Verification items for the finished model (mm, model axes). Face numbers are marked on the shaded views. A direction names the side the tool comes from. Coordinates: 2 decimals unless noted, no trailing zeros. Write each loop counter-clockwise with the first axis right and the second up, starting at its lowest first coordinate (ties: lowest second). Pieces come first, ordered by that corner, then holes. Notation, with made-up numbers: (8, -12.75) -> (12, -12.75) arc R14 cw to (12, 7.25) -> close; hole circle Ø7 at (64, -19). An arc over 180 degrees is marked (long way). Answer in a Markdown table with one row per item.
```python
from build123d import *

# Parameters (mm, degrees)
SKETCH1_R           = 40
SKETCH1_R_2         = 6
SKETCH1_W           = 6.8
SKETCH1_H           = 1.7
BOSS_EXTRUDE1_DEPTH = 10
SKETCH3_R           = 40
SKETCH3_W           = 30
SKETCH3_H           = 46.499999994
BOSS_EXTRUDE3_DEPTH = 25
CUT_EXTRUDE1_START  = -35
CUT_EXTRUDE1_DEPTH  = 35
SKETCH5_R           = 2.55
CUT_EXTRUDE2_DEPTH  = 5
CUT_EXTRUDE3_DEPTH  = 25
SKETCH8_W           = 22
SKETCH8_H           = 8
CUT_EXTRUDE4_DEPTH  = 22


with BuildPart() as part:
    # Sketch1 → Boss-Extrude1 (new body)
    with BuildSketch(Plane.XY):
        with Locations((0, 222.499999997)):
            Circle(SKETCH1_R)
        with Locations((0, 234.5)):
            Circle(SKETCH1_R_2, mode=Mode.SUBTRACT)
        with Locations((0, 200.1)):
            Rectangle(SKETCH1_W, SKETCH1_H, mode=Mode.SUBTRACT)
        with BuildLine():
            ThreePointArc((11, 243.75), (9.75, 242.5), (11, 241.25))
            ThreePointArc((11, 241.25), (12.25, 242.5), (11, 243.75))
        make_face(mode=Mode.SUBTRACT)
        with BuildLine():
            ThreePointArc((-11, 241.25), (-9.75, 242.5), (-11, 243.75))
            ThreePointArc((-11, 243.75), (-12.25, 242.5), (-11, 241.25))
        make_face(mode=Mode.SUBTRACT)
        with BuildLine():
            ThreePointArc((11, 201.25), (12.25, 202.5), (11, 203.75))
            ThreePointArc((11, 203.75), (9.75, 202.5), (11, 201.25))
        make_face(mode=Mode.SUBTRACT)
        with BuildLine():
            ThreePointArc((-11, 201.25), (-9.75, 202.5), (-11, 203.75))
            ThreePointArc((-11, 203.75), (-12.25, 202.5), (-11, 201.25))
        make_face(mode=Mode.SUBTRACT)
    extrude(amount=BOSS_EXTRUDE1_DEPTH)

    # Sketch3 → Boss-Extrude3 (add)
    with BuildSketch(Plane.XY.offset(10)):
        with Locations((0, 222.499999997)):
            Circle(SKETCH3_R)
        with Locations((0, 222.499999997)):
            Rectangle(SKETCH3_W, SKETCH3_H, mode=Mode.SUBTRACT)
    extrude(amount=BOSS_EXTRUDE3_DEPTH)

    # Sketch4 → Cut-Extrude1 (cut)
    with BuildSketch(Plane.XY.offset(35).offset(CUT_EXTRUDE1_START)):
        with BuildLine():
            ThreePointArc((40, 222.499999997), (38.912456167, 231.763949212), (35.708962247, 240.524150885))
            ThreePointArc((35.708962247, 240.524150885), (31.77566454, 233.14486234), (30.74061322, 224.84706751))
            ThreePointArc((30.74061322, 224.84706751), (30.809531665, 222.499999997), (30.74061322, 220.152932484))
            ThreePointArc((30.74061322, 220.152932484), (31.77566454, 211.855137653), (35.708962247, 204.475849108))
            ThreePointArc((35.708962247, 204.475849108), (38.912456167, 213.236050782), (40, 222.499999997))
        make_face()
        with BuildLine():
            ThreePointArc((-2.347067513, 191.759386777), (-10.644862344, 190.724335457), (-18.024150889, 186.79103775))
            ThreePointArc((-18.024150889, 186.79103775), (0, 182.499999997), (18.024150889, 186.79103775))
            ThreePointArc((18.024150889, 186.79103775), (10.644862344, 190.724335457), (2.347067513, 191.759386777))
            ThreePointArc((2.347067513, 191.759386777), (0, 191.690468331), (-2.347067513, 191.759386777))
        make_face()
        with BuildLine():
            ThreePointArc((18.024150889, 258.208962244), (0, 262.499999997), (-18.024150889, 258.208962244))
            ThreePointArc((-18.024150889, 258.208962244), (-10.644862344, 254.275664537), (-2.347067513, 253.240613217))
            ThreePointArc((-2.347067513, 253.240613217), (0, 253.309531662), (2.347067513, 253.240613217))
            ThreePointArc((2.347067513, 253.240613217), (10.644862344, 254.275664537), (18.024150889, 258.208962244))
        make_face()
        with BuildLine():
            ThreePointArc((-30.74061322, 220.152932484), (-30.809531665, 222.499999997), (-30.74061322, 224.84706751))
            ThreePointArc((-30.74061322, 224.84706751), (-31.77566454, 233.14486234), (-35.708962247, 240.524150885))
            ThreePointArc((-35.708962247, 240.524150885), (-40, 222.499999997), (-35.708962247, 204.475849108))
            ThreePointArc((-35.708962247, 204.475849108), (-31.77566454, 211.855137653), (-30.74061322, 220.152932484))
        make_face()
    extrude(amount=CUT_EXTRUDE1_DEPTH, mode=Mode.SUBTRACT)

    # Sketch5 → Cut-Extrude2 (cut)
    with BuildSketch(Plane.XY.offset(35)):
        with Locations((-22.627416998, 245.127416995)):
            Circle(SKETCH5_R)
        with Locations(Location((22.627416998, 245.127416995, 0), (0, 0, 180))):
            Circle(SKETCH5_R)
        with Locations((22.627416998, 199.872582999)):
            Circle(SKETCH5_R)
        with Locations(Location((-22.627416998, 199.872582999, 0), (0, 0, 180))):
            Circle(SKETCH5_R)
    extrude(amount=-CUT_EXTRUDE2_DEPTH, mode=Mode.SUBTRACT)

    # Sketch6 → Cut-Extrude3 (cut)
    with BuildSketch(Plane.XY.offset(35)):
        with BuildLine():
            Line((-15, 218.499999997), (-15, 226.499999997))
            ThreePointArc((-15, 226.499999997), (-19, 222.499999997), (-15, 218.499999997))
        make_face()
        with BuildLine():
            Line((15, 218.499999997), (15, 226.499999997))
            ThreePointArc((15, 226.499999997), (19, 222.499999997), (15, 218.499999997))
        make_face()
    extrude(amount=-CUT_EXTRUDE3_DEPTH, mode=Mode.SUBTRACT)

    # Sketch8 → Cut-Extrude4 (cut)
    with BuildSketch(Plane(origin=(-15, 0, 0), x_dir=(0, 0, -1), z_dir=(1, 0, 0))):
        with Locations((-11, 222.499999997)):
            Rectangle(SKETCH8_W, SKETCH8_H)
    extrude(amount=-CUT_EXTRUDE4_DEPTH, mode=Mode.SUBTRACT)


solid = part.part
```
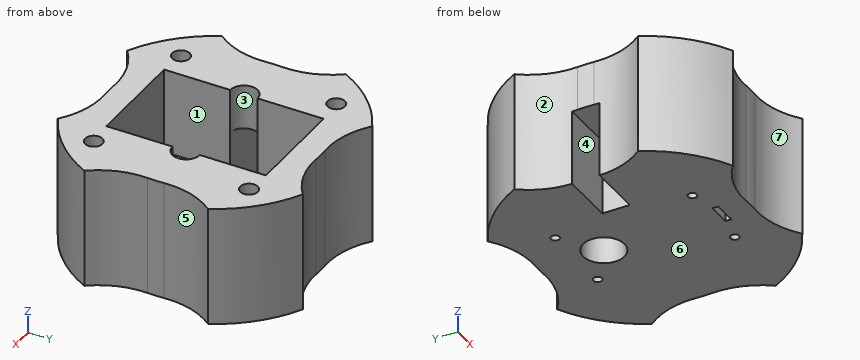
1. Go/stop test with flat-tipped pins: pin 1 (15.5 mm diameter, centred on y = 213, z = 24.5, fed in from +X); pin 2 (6 mm diameter, centred on y = 202.5, z = 20.5, fed in from +X); pin 3 (1.9 mm diameter, centred on y = 200, z = 5.5, fed in from +X). Record where each tip stops, or that it passes through.
Findings below:
| item | result |
|---|---|
| pin 1 | stops at x = 35.12 |
| pin 2 | stops at x = 35.71 |
| pin 3 | stops at x = 33.7 |
2. Sectioned sample at D-D, the plane z = 14.5. Record the cut outline in (x, y).
Findings below:
| item | result |
|---|---|
| outline | (-35.71, 204.48) arc R40 ccw to (-18.02, 186.79) arc R23 cw to (-2.35, 191.76) arc R40 ccw to (2.35, 191.76) arc R23 cw to (18.02, 186.79) arc R40 ccw to (35.71, 204.48) arc R23 cw to (30.74, 220.15) arc R40 ccw to (30.74, 224.85) arc R23 cw to (35.71, 240.52) arc R40 ccw to (18.02, 258.21) arc R23 cw to (2.35, 253.24) arc R40 ccw to (-2.35, 253.24) arc R23 cw to (-18.02, 258.21) arc R40 ccw to (-35.71, 240.52) arc R23 cw to (-30.7, 226.5) -> (-15, 226.5) -> (-15, 245.75) -> (15, 245.75) -> (15, 226.5) arc R4 cw to (15, 218.5) -> (15, 199.25) -> (-15, 199.25) -> (-15, 218.5) -> (-30.7, 218.5) arc R23 cw to start |
3. Sectioned sample at B-B, the plane z = 29. Record the cut outline in (x, y).
Findings below:
| item | result |
|---|---|
| outline | (-35.71, 204.48) arc R40 ccw to (-18.02, 186.79) arc R23 cw to (-2.35, 191.76) arc R40 ccw to (2.35, 191.76) arc R23 cw to (18.02, 186.79) arc R40 ccw to (35.71, 204.48) arc R23 cw to (30.74, 220.15) arc R40 ccw to (30.74, 224.85) arc R23 cw to (35.71, 240.52) arc R40 ccw to (18.02, 258.21) arc R23 cw to (2.35, 253.24) arc R40 ccw to (-2.35, 253.24) arc R23 cw to (-18.02, 258.21) arc R40 ccw to (-35.71, 240.52) arc R23 cw to (-30.74, 224.85) arc R40 ccw to (-30.74, 220.15) arc R23 cw to start; hole (-15, 199.25) -> (15, 199.25) -> (15, 218.5) arc R4 ccw to (15, 226.5) -> (15, 245.75) -> (-15, 245.75) -> (-15, 226.5) arc R4 ccw to (-15, 218.5) -> close |
4. Sectioned sample at A-A, the plane x = 0. Record the cut outline in (y, z), and give its area (3 significant figures).
Findings below:
| item | result |
|---|---|
| outline | (191.69, 0) -> (199.25, 0) -> (199.25, 35) -> (191.69, 35) -> close; (200.95, 0) -> (228.5, 0) -> (228.5, 10) -> (200.95, 10) -> close; (240.5, 0) -> (253.31, 0) -> (253.31, 35) -> (245.75, 35) -> (245.75, 10) -> (240.5, 10) -> close |
| area | 857 mm² |
5. Material ranges on probe 1 along X at (y, z) = (202.5, 2.5); probe 2 along X at (y, z) = (240.5, 26.5); probe 3 along X at (y, z) = (243, 16), recorded low to high. Write a range as from..to.
Findings below:
| item | result |
|---|---|
| probe 1 | x = -34.64..-12.25, -9.75..9.75, 12.25..34.64 |
| probe 2 | x = -35.69..-15, 15..35.69 |
| probe 3 | x = -34.35..-15, 15..34.35 |
6. Release check for a two-part mould opening along Y. For the marked faces 5, 6 and 7 record: released by +Y, released by -Y, zero draft, split by the parting line, or undercut.
Findings below:
| item | result |
|---|---|
| face 5 | undercut |
| face 6 | zero draft |
| face 7 | released by -Y |
7. Access from +Z, -Z, +X, -X, +Y, -Y to the whole of each face (thin tool, end or side, straight path). Record for the marked faces 1, 2, 3 and 4.
Findings below:
| item | result |
|---|---|
| face 1 | +Z |
| face 2 | +Z, -Z, -X |
| face 3 | +Z, -Z |
| face 4 | -Z, -X |
8. Sectioned sample at C-C, the plane y = 222.5. Record the cut outline in (x, z).
Findings below:
| item | result |
|---|---|
| outline | (-30.81, 22) -> (-19, 22) -> (-19, 35) -> (-30.81, 35) -> close; (-15, 0) -> (30.81, 0) -> (30.81, 35) -> (19, 35) -> (19, 10) -> (-15, 10) -> close |
